Geometry: final body of the model. Coordinates: model frame, mm. Face numbers are marked on the shaded views. A direction names the side the tool comes from. Give positions to 0.01 mm unless a question says otherwise; leave off trailing zeros. Write each loop counter-clockwise with the first axis right and the second up, starting at its lowest first coordinate (ties: lowest second). Pieces come first, ordered by that corner, then holes.
Q1. Section C-C (z = -25). Return the cut outline in (x, y).
Q2. Pin query (flat end, axial travel): pin 1 Ø3 at (x, z) = (37.5, 21) entering from +Y; pin 2 Ø13.5 at (x, y) = (-46.5, -37.5) entering from -Z; pin 3 Ø13 at (x, z) = (35.19, -22.89) entering from -Y; pin 4 Ø12 at (x, z) = (-51.5, -14) entering from -Y. Return the tip coordinate at first contact, or that it passes through.
Q3. Reachability of the marked faces 1, 2 and 3 from +Z, -Z, +X, -X, +Y, -Y: full face, straight path, thin tool, end or side. Return the list, or none.
Q4. Line query: line 1 (X direction, y = -34, z = 3); line 2 (Y direction, x = 35, z = 22); line 3 (X direction, y = -3, z = 32.5). Output: solid intervals per line, ascending.
Q5. Section D-D (x = 11). Return the cut outline in (y, z).
Q6. Section B-B (z = 5). Return the cut outline in (x, y).
from build123d import *
from build123d.topology import SkipClean

# Parameters (mm, degrees)
SKETCH1_W           = 135
SKETCH1_H           = 93
SKETCH1_R           = 3
BOSS_EXTRUDE1_DEPTH = 7
SKETCH2_R           = 4
BOSS_EXTRUDE2_DEPTH = 39
FILLET1_R           = 10
SKETCH3_R           = 8
BOSS_EXTRUDE3_DEPTH = 8
SKETCH4_W           = 13.352525021
SKETCH4_H           = 5.289406047
BOSS_EXTRUDE4_DEPTH = 23
SKETCH5_R           = 4
CUT_EXTRUDE1_DEPTH  = 23
BOSS_EXTRUDE5_START = 4
SKETCH6_R           = 8.5
SKETCH6_R_2         = 6
SKETCH6_R_3         = 3
BOSS_EXTRUDE5_DEPTH = 4


with BuildPart() as part:
    # Sketch1 → Boss-Extrude1 (new body)
    with BuildSketch(Plane.XY):
        Rectangle(SKETCH1_W, SKETCH1_H)
        with Locations((-49.35483871, 34)):
            Circle(SKETCH1_R, mode=Mode.SUBTRACT)
        with Locations((49.35483871, 34)):
            Circle(SKETCH1_R, mode=Mode.SUBTRACT)
        with Locations((-49.35483871, -34)):
            Circle(SKETCH1_R, mode=Mode.SUBTRACT)
        with Locations((49.35483871, -34)):
            Circle(SKETCH1_R, mode=Mode.SUBTRACT)
    extrude(amount=BOSS_EXTRUDE1_DEPTH)

    # Sketch2 → Boss-Extrude2 (add)
    with BuildSketch(Plane.XY.offset(7)):
        with BuildLine():
            Line((-35.5, 19), (35.5, 19))
            ThreePointArc((35.5, 19), (54.5, 0), (35.5, -19))
            Line((35.5, -19), (-35.5, -19))
            ThreePointArc((-35.5, -19), (-54.5, 0), (-35.5, 19))
        make_face()
        with Locations((-35.5, 0)):
            Circle(SKETCH2_R, mode=Mode.SUBTRACT)
        with Locations((35.5, 0)):
            Circle(SKETCH2_R, mode=Mode.SUBTRACT)
    extrude(amount=BOSS_EXTRUDE2_DEPTH)

    # Fillet1
    fillet1_edges = [part.edges().sort_by_distance(p)[0] for p in [
        (-67.5, -46.5, 3.5),
        (-67.5, 46.5, 3.5),
        (67.5, 46.5, 3.5),
        (67.5, -46.5, 3.5),
    ]]
    fillet(fillet1_edges, radius=FILLET1_R)

    # Sketch3 → Boss-Extrude3 (add)
    with BuildSketch(Plane(origin=(0, 0, 0), x_dir=(-1, 0, 0), z_dir=(0, 0, -1))):
        with Locations(Location((-35.5, 0, 0), (0, 0, 180))):
            Circle(SKETCH3_R)
        with Locations(Location((35.5, 0, 0), (0, 0, 180))):
            Circle(SKETCH3_R)
    extrude(amount=BOSS_EXTRUDE3_DEPTH)

    # Sketch4 → Boss-Extrude4 (add)
    with BuildSketch(Plane(origin=(0, 0, -8), x_dir=(-1, 0, 0), z_dir=(0, 0, -1))):
        with Locations((-35.191522183, -0.266454552)):
            Rectangle(SKETCH4_W, SKETCH4_H)
        with Locations((35.191522183, -0.266454552)):
            Rectangle(SKETCH4_W, SKETCH4_H)
    extrude(amount=BOSS_EXTRUDE4_DEPTH)

    # Sketch5 → Cut-Extrude1 (cut)
    with BuildSketch(Plane(origin=(0, 2.378248472, 0), x_dir=(1, 0, 0), z_dir=(0, 1, 0))):
        with Locations(Location((35.191522184, 22.89088314, 0), (0, 0, 270))):
            Circle(SKETCH5_R)
        with Locations(Location((-35.191522184, 22.89088314, 0), (0, 0, 270))):
            Circle(SKETCH5_R)
    extrude(amount=-CUT_EXTRUDE1_DEPTH, mode=Mode.SUBTRACT)

    # Sketch6 → Boss-Extrude5 (add)
    # profile 1 of 4: a face of its own
    with SkipClean():  # the faces are left unmerged after this step: merging them gives an invalid solid
        with BuildSketch(Plane(origin=(0, 0, 0), x_dir=(-1, 0, 0), z_dir=(0, 0, -1)).offset(BOSS_EXTRUDE5_START)):
            with Locations(Location((-49.35483871, 34, 0), (0, 0, 180))):
                Circle(SKETCH6_R)
            with Locations((-49.35483871, 34)):
                Circle(SKETCH6_R_2, mode=Mode.SUBTRACT)
        # profile 2 of 4: a face of its own
        with BuildSketch(Plane(origin=(0, 0, 0), x_dir=(-1, 0, 0), z_dir=(0, 0, -1)).offset(BOSS_EXTRUDE5_START)):
            with Locations((-49.35483871, -34)):
                Circle(SKETCH6_R)
            with Locations((-49.35483871, -34)):
                Circle(SKETCH6_R_3, mode=Mode.SUBTRACT)
        # profile 3 of 4: a face of its own
        with BuildSketch(Plane(origin=(0, 0, 0), x_dir=(-1, 0, 0), z_dir=(0, 0, -1)).offset(BOSS_EXTRUDE5_START)):
            with Locations(Location((49.35483871, -34, 0), (0, 0, 180))):
                Circle(SKETCH6_R)
            with Locations((49.35483871, -34)):
                Circle(SKETCH6_R_3, mode=Mode.SUBTRACT)
        # profile 4 of 4: a face of its own
        with BuildSketch(Plane(origin=(0, 0, 0), x_dir=(-1, 0, 0), z_dir=(0, 0, -1)).offset(BOSS_EXTRUDE5_START)):
            with Locations((49.35483871, 34)):
                Circle(SKETCH6_R)
            with Locations((49.35483871, 34)):
                Circle(SKETCH6_R_3, mode=Mode.SUBTRACT)
        extrude(amount=-BOSS_EXTRUDE5_DEPTH)


solid = part.part
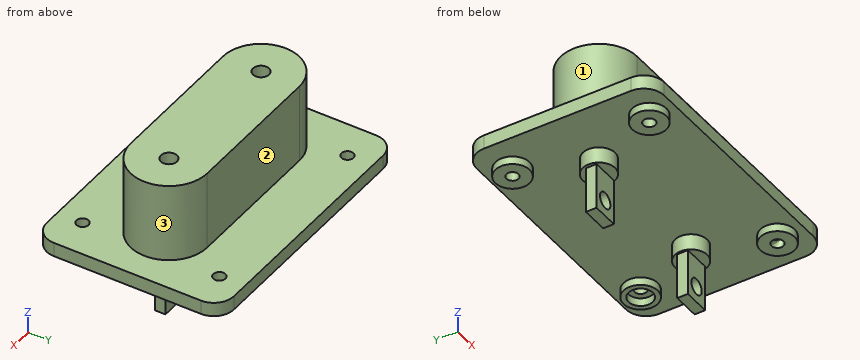
Computed:
1. outline: (-41.87, -2.91) - (-38.59, -2.91) - (-38.59, 2.38) - (-41.87, 2.38) - close; (-31.79, -2.91) - (-28.52, -2.91) - (-28.52, 2.38) - (-31.79, 2.38) - close; (28.52, -2.91) - (31.79, -2.91) - (31.79, 2.38) - (28.52, 2.38) - close; (38.59, -2.91) - (41.87, -2.91) - (41.87, 2.38) - (38.59, 2.38) - close
2. pin 1: stops at y = 18.99
2. pin 2: stops at z = -4
2. pin 3: stops at y = -2.91
2. pin 4: passes through
3. face 1: +Z, -X
3. face 2: +Z, +X, -X, +Y
3. face 3: +Z, +X
4. line 1: x = -67.5 to -52.35, -46.35 to 46.35, 52.35 to 67.5
4. line 2: y = -19 to -3.97, 3.97 to 19
4. line 3: x = -54.26 to -38.15, -32.85 to 32.85, 38.15 to 54.26
5. outline: (-46.5, 0) - (46.5, 0) - (46.5, 7) - (19, 7) - (19, 46) - (-19, 46) - (-19, 7) - (-46.5, 7) - close
6. outline: (-67.5, -36.5) arc R10 ccw to (-57.5, -46.5) - (57.5, -46.5) arc R10 ccw to (67.5, -36.5) - (67.5, 36.5) arc R10 ccw to (57.5, 46.5) - (-57.5, 46.5) arc R10 ccw to (-67.5, 36.5) - close; hole circle Ø6 at (-49.35, -34); hole circle Ø6 at (-49.35, 34); hole circle Ø6 at (49.35, -34); hole circle Ø6 at (49.35, 34)
